Here's how the part is built. I have some questions about the finished solid (model axes, mm). Face numbers are marked on the shaded views. Give positions to 0.01 mm unless a question says otherwise; leave off trailing zeros. Order: outer loops, then holes, each group sorted by start corner. A loop starts at its lowest first (then second) coordinate and runs counter-clockwise, first axis right, second up. Notation, with made-up numbers: M 32,73.25 L 76,73.25 A23 ccw 76,82.25 Z; hole C -22,-30 d11. An arc over 180 degrees is marked long. Use one line per item in the form item = value.
from build123d import *

# Parameters (mm, degrees)
SKETCH1_W           = 30
SKETCH1_H           = 34
BOSS_EXTRUDE1_DEPTH = 22
CUT_EXTRUDE1_REACH  = 52.398
SKETCH2_R           = 4
SKETCH3_R           = 2.5
CUT_EXTRUDE2_DEPTH  = 22


with BuildPart() as part:
    # Sketch1 → Boss-Extrude1 (new body)
    with BuildSketch(Plane(origin=(0, 0, 0), x_dir=(1, 0, 0), z_dir=(0, 1, 0))):
        with Locations((15, 17)):
            Rectangle(SKETCH1_W, SKETCH1_H)
    extrude(amount=BOSS_EXTRUDE1_DEPTH)

    # Sketch2 → Cut-Extrude1 (cut, up to next)
    with BuildSketch(Plane.XY, mode=Mode.PRIVATE) as cut_extrude1_sk1:
        with Locations((14.820555819, 11)):
            Circle(SKETCH2_R)
    cut_extrude1_tool1 = extrude(cut_extrude1_sk1.sketch, amount=-CUT_EXTRUDE1_REACH, mode=Mode.PRIVATE) & part.part
    # Sketch2 → Cut-Extrude1 (cut, up to next)
    with BuildSketch(Plane.XY, mode=Mode.PRIVATE) as cut_extrude1_sk2:
        Polygon((0, 14), (7.5, 22), (0, 22), align=None)
    cut_extrude1_tool2 = extrude(cut_extrude1_sk2.sketch, amount=-CUT_EXTRUDE1_REACH, mode=Mode.PRIVATE) & part.part
    # Sketch2 → Cut-Extrude1 (cut, up to next)
    with BuildSketch(Plane.XY, mode=Mode.PRIVATE) as cut_extrude1_sk3:
        Polygon((30, 14), (22.5, 22), (30, 22), align=None)
    cut_extrude1_tool3 = extrude(cut_extrude1_sk3.sketch, amount=-CUT_EXTRUDE1_REACH, mode=Mode.PRIVATE) & part.part
    add(cut_extrude1_tool1.solids().sort_by_distance((14.820556, 11, 0))[0], mode=Mode.SUBTRACT)
    add(cut_extrude1_tool2.solids().sort_by_distance((2.5, 19.333333, 0))[0], mode=Mode.SUBTRACT)
    add(cut_extrude1_tool3.solids().sort_by_distance((27.5, 19.333333, 0))[0], mode=Mode.SUBTRACT)

    # Sketch3 → Cut-Extrude2 (cut)
    with BuildSketch(Plane.XZ):
        with Locations(Location((6, -8, 0), (0, 0, 270))):
            Circle(SKETCH3_R)
        with Locations(Location((24, -8, 0), (0, 0, 270))):
            Circle(SKETCH3_R)
        with Locations(Location((24, -26, 0), (0, 0, 270))):
            Circle(SKETCH3_R)
        with Locations(Location((6, -26, 0), (0, 0, 270))):
            Circle(SKETCH3_R)
    extrude(amount=-CUT_EXTRUDE2_DEPTH, mode=Mode.SUBTRACT)


solid = part.part
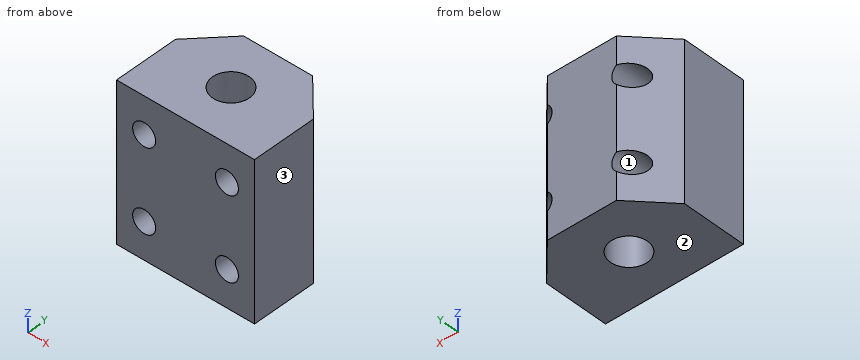
Q1. I need wall thicknesses on L1, parallel to Z at x = 24, y = 6.5; L2, parallel to Z at x = 22, y = 13.5; L3, parallel to X at y = 11.25, z = -22. Which ranges of each line are inside material? Lowest first, please.
Found:
L1 = -34 to -28.5, -23.5 to -10.5, -5.5 to 0
L2 = -34 to -27.5, -24.5 to -9.5, -6.5 to 0
L3 = 0 to 10.83, 18.81 to 30
Q2. I want a section at B-B on x = 6. Write out the boundary of the cut face in (y, z), then the cut area to 3 significant figures.
Found:
outline = M 0,-34 L 20.4,-34 L 20.4,-28.5 L 0,-28.5 Z; M 0,-23.5 L 20.4,-23.5 L 20.4,-10.5 L 0,-10.5 Z; M 0,-5.5 L 20.4,-5.5 L 20.4,0 L 0,0 Z
area = 490 mm²
Q3. I want a section at D-D on z = -13. Write out the boundary of the cut face in (x, y), then the cut area to 3 significant figures.
Found:
outline = M 0,0 L 30,0 L 30,14 L 22.5,22 L 7.5,22 L 0,14 Z; hole C 14.82,11 d8
area = 550 mm²
Q4. Thinking about a two-plate mould opening in Z: for the marked faces 1, 2 and 3, which applies, +Z half, -Z half, draft (parallel to the pull), parting line (faces both ways), or undercut?
Found:
face_1 = undercut
face_2 = -Z half
face_3 = draft
Q5. I'm going to push a flat-ended pin straight in: pin 1 Ø2 at (y, z) = (16.5, -12) entering from -X. Where does the tip first touch, or does it pass through?
Found:
pin_1 = 1.41
Q6. I want a section at C-C on z = -25.5. Write out the boundary of the cut face in (x, y), then the cut area to 3 significant figures.
Found:
outline = M 0,0 L 3.55,0 L 3.55,17.79 L 0,14 Z; M 8.45,0 L 21.55,0 L 21.55,22 L 8.45,22 Z; M 26.45,0 L 30,0 L 30,14 L 26.45,17.79 Z; hole C 14.82,11 d8
area = 351 mm²
Q7. I want a section at A-A on y = 11. Write out the boundary of the cut face in (x, z).
Found:
outline = M 0,-34 L 10.82,-34 L 10.82,0 L 0,0 Z; M 18.82,-34 L 30,-34 L 30,0 L 18.82,0 Z; hole C 6,-26 d5; hole C 6,-8 d5; hole C 24,-26 d5; hole C 24,-8 d5
